Autodesk Inventor part; units mm, degrees
ref_plane "YZ Plane" through (0, 0, 0) normal (1, 0, 0) x (0, 1, 0)
ref_plane "XZ Plane" through (0, 0, 0) normal (0, 1, 0) x (-1, 0, 0)
ref_plane "XY Plane" through (0, 0, 0) normal (0, 0, 1) x (1, 0, 0)
sketch "Sketch1" plane through (0, 0, 0) normal (0, 0, 1) x (1, 0, 0)
  circle A0 centre (0, 0) radius 2.5
  circle A1 centre (15.5, 15.5) radius 1.6
  line L0 (-19.231, 2.5) -> (-12.5, 2.5)
  line L1 (-12.5, 2.5) -> (-12.5, -2.5)
  line L2 (-12.5, -2.5) -> (-19.231, -2.5)
  line L3 (-19.231, -2.5) -> (-19.231, 2.5)
  line L4 (20, 7.5) -> (26.731, 7.5)
  line L5 (26.731, 7.5) -> (26.731, -7.5)
  line L6 (26.731, -7.5) -> (20, -7.5)
  line L7 (20, -7.5) -> (20, 7.5)
  line L8 (-30.769, 27.5) -> (29.231, 27.5)
  line L9 (29.231, 27.5) -> (29.231, -29.231)
  line L10 (29.231, -29.231) -> (-30.769, -29.231)
  line L11 (-30.769, -29.231) -> (-30.769, 27.5)
  line L12 (4.231, -20) -> (19.231, -20)
  line L13 (19.231, -20) -> (19.231, -26.731)
  line L14 (19.231, -26.731) -> (4.231, -26.731)
  line L15 (4.231, -26.731) -> (4.231, -20)
  line L16 (-29.162, 2.5) -> (-22.431, 2.5)
  line L17 (-22.431, 2.5) -> (-22.431, -2.5)
  line L18 (-22.431, -2.5) -> (-29.162, -2.5)
  line L19 (-29.162, -2.5) -> (-29.162, 2.5)
  line L20 (-20.769, -20) -> (-5.769, -20)
  line L21 (-5.769, -20) -> (-5.769, -26.731)
  line L22 (-5.769, -26.731) -> (-20.769, -26.731)
  line L23 (-20.769, -26.731) -> (-20.769, -20)
  line L24 (-10, -17.5) -> (-10, 17.5)
  line L25 (-10, 17.5) -> (10, 17.5)
  line L26 (-10, -17.5) -> (17.5, -17.5)
  line L27 (17.5, -17.5) -> (17.5, 10)
  arc A2 (10, 17.5) -> (17.5, 10) centre (17.5, 17.5) ccw
  line L28 (-10, -17.5) -> (-6, 0)
  line L29 (6, 0) -> (17.5, -17.5)
  arc A3 (6, 0) -> (-6, 0) centre (0, 0) ccw
  circle A4 centre (-15.5, -15.5) radius 1.6
  point P0 (-12.5, 0)
  point P1 (20, 0)
  dimension "d0" = 5
  dimension "d6" = 32.5
  dimension "d7" = 20
  dimension "d8" = 5
  dimension "d9" = 6.731
  dimension "d13" = 20
  dimension "d17" = 2.5
  dimension "d18" = 20
  dimension "d19" = 2.5
  dimension "d20" = 3.2
  dimension "d25" = 15
  dimension "d26" = 10
  dimension "d28" = 60
  dimension "d29" = 10
  dimension "d30" = 15.5
  dimension "d31" = 15.5
  dimension "d32" = 3.2
  dimension "d33" = 2.5
  dimension "d34" = 2.5
  dimension "d35" = 2.5
  dimension "d36" = 7.5
  dimension "d37" = 6
  dimension "d39" = 35
  dimension "d40" = 15.5
  dimension "d41" = 15.5
extrude "Extrusion2" add sketch "Sketch1" along normal blind 6.731 contours L8 L9 L10 L11
fillet "Fillet2" radius 5 4 edges at (29.231, 27.5, 3.3655) (29.231, -29.231, 3.3655) (-30.769, -29.231, 3.3655) (-30.769, 27.5, 3.3655)
fillet "Fillet2" radius 1.5875 5 edges at (-10, -17.5, 3.3655) (17.5, -17.5, 3.3655) (17.5, 10, 3.3655) (10, 17.5, 3.3655) (-10, 17.5, 3.3655)
equation "\"d9\" = THICKB"
equation "\"d29\" = d26"
equation "\"d22\" = THICKB"
equation "\"THICKA\" = 3.175"
equation "\"THICKB\" = 6.731"
equation "\"THICKC\" = 12.7"
equation "\"BALLDIA\" = 12"
equation "\"MAGDIA\" = 9.5"
properties part number "Air2D_Side_Face"
Check sheet for the modelled part. Datum: model origin and axes. Units: mm. A direction names the side the tool comes from. Round coordinates to 2 decimals unless told otherwise and drop trailing zeros. Order: outer loops, then holes, each group sorted by start corner. A loop starts at its lowest first (then second) coordinate and runs counter-clockwise, first axis right, second up. Notation, with made-up numbers: (85.25, -3.5) - (141.25, -3.5) arc R25 ccw to (141.25, 18.5) - close; hole circle Ø3 at (-20, 45). An arc over 180 degrees is marked (long way). Answer as CSV lines item,"result". Start each with the question number.
1) Draft check along X on faces 3 (the face through (17.14, 9.56, 3.41)), 4 (the face through (-5.769, -23, 3)), 5 (the face through (-15, 6, 0)), 6 (the face through (-29.27, 26.07, 3.41)). Enter one of: +X half, -X half, draft (parallel to the pull), parting line (faces both ways), or undercut.
2) Section check B-B (x = -20). Record the cut outline in (y, z), then the cut area to 3 significant figures.
3) Section check D-D (y = 12). Record the cut outline in (x, z).
4) Section check A-A (y = -6.5). Record the cut outline in (x, z).
5) Scan lines: probe 1 along Y at (x, z) = (8.5, 5.75); probe 2 along X at (y, z) = (2, 3.5); probe 3 along X at (y, z) = (3.5, 1.75). Record each from-to range of solid material in increasing order.
6) Depth check by flat-ended pin: pin 1 (4 mm diameter, centred on x = 6.5, y = 19.5, fed in from -Z). Enter the tip coordinate at first touch or a pass-through.
7) Tool access check on faces 1 (the face through (-22.431, 0, 3)), 2 (the face through (-30.769, -1, 3)). Record the directions out of +Z, -Z, +X, -X, +Y, -Y that give a thin tool (end or side, any length) a straight path to the whole face; none if there is none.
8) Section check C-C (x = 15). Record the cut outline in (y, z), then the cut area to 3 significant figures.
Determined:
1,face 3,"undercut"
1,face 4,"undercut"
1,face 5,"draft"
1,face 6,"-X half"
2,outline,"(-29.23, 0) - (-26.73, 0) - (-26.73, 6.73) - (-29.23, 6.73) - close; (-20, 0) - (27.5, 0) - (27.5, 6.73) - (-20, 6.73) - close"
2,area,"337 mm^2"
3,outline,"(-30.77, 0) - (-10, 0) - (-10, 6.73) - (-30.77, 6.73) - close; (12.4, 0) - (29.23, 0) - (29.23, 6.73) - (12.4, 6.73) - close"
4,outline,"(-30.77, 0) - (-10, 0) - (-10, 6.73) - (-30.77, 6.73) - close; (17.5, 0) - (20, 0) - (20, 6.73) - (17.5, 6.73) - close; (26.73, 0) - (29.23, 0) - (29.23, 6.73) - (26.73, 6.73) - close"
5,probe 1,"-29.23 to -26.73, -20 to -17.5, 17.5 to 27.5"
5,probe 2,"-30.77 to -29.16, -22.43 to -19.23, -12.5 to -10, 17.5 to 20, 26.73 to 29.23"
5,probe 3,"-30.77 to -10, 17.5 to 20, 26.73 to 29.23"
6,pin 1,"z = 0"
7,face 1,"+Z, -Z"
7,face 2,"+Z, -Z, -X, +Y, -Y"
8,outline,"(-29.23, 0) - (-26.73, 0) - (-26.73, 6.73) - (-29.23, 6.73) - close; (-20, 0) - (-17.5, 0) - (-17.5, 6.73) - (-20, 6.73) - close; (10.43, 0) - (13.98, 0) - (13.98, 6.73) - (10.43, 6.73) - close; (17.02, 0) - (27.5, 0) - (27.5, 6.73) - (17.02, 6.73) - close"
8,area,"128 mm^2"
